from build123d import *

# Parameters (mm, degrees)
F1_R     = 63.5
F2_R     = 76.2
F4_R     = 26.2509
F5_DEPTH = 355.6
F6_R     = 25.4
F7_DEPTH = 95.25


with BuildPart() as f3:
    # F1 (on Top) → F3 section 0
    with BuildSketch(Plane.XY):
        Circle(F1_R)
    # F2 (on offset) → F3 section 1
    with BuildSketch(Plane.XY.offset(228.6)):
        Circle(F2_R)
    loft()

    # F4 (on Front) → F5 (join)
    with BuildSketch(Plane.XZ):
        with Locations((0, 151.5491)):
            Circle(F4_R)
    extrude(amount=F5_DEPTH)

    # F6 (on Front) → F7 (join)
    with BuildSketch(Plane.XZ):
        with Locations((0, 76.2)):
            Circle(F6_R)
    extrude(amount=-F7_DEPTH)


solid = f3.part
For this review, take the finished solid that the model builds, in its own axes (mm). A direction names the side the tool comes from. Give positions to 0.01 mm unless a question says otherwise; leave off trailing zeros. Order: outer loops, then holes, each group sorted by start corner. A loop starts at its lowest first (then second) coordinate and runs counter-clockwise, first axis right, second up. Notation, with made-up numbers: M 29,17 L 62,17 A15 ccw 62,36 Z; hole C -12.75,49.25 d4. An arc over 180 degrees is marked long. Answer in a Markdown table with one row per item. Add a question column.
(1) Consider section A-A on x = 0. State the section outline as (y, z) points, and give its area (3 significant figures).
(2) Consider section D-D on z = 86. State the section outline as (x, y) points, and give its area (3 significant figures).
(3) Consider section B-B on z = 111.5. State the section outline as (x, y) points.
(4) For faces 1 (the face through (-5.691, -209.179, 125.922)), 2 (the face through (0, -355.6, 152)), 3 (the face through (-5.506, 78.717, 51.404)), list the 3-axis set-ups (+Z, -Z, +X, -X, +Y, -Y) from which the entire face can be reached by the end or side of a thin tool; tool diameter is ignored.
(5) Wall thickness on probe 1 along Y at (x, z) = (35, 163); probe 2 along X at (y, z) = (-86, 157); probe 3 along Y at (x, z) = (27, 32): over which ranges is each line inside the solid? List them lowest first. Write a range as [from, to].
(6) Consider section C-C on y = -267. State the section outline as (x, z) points.
(7) For pin 1 (1 mm diameter, centred on x = 36, z = 40.5, fed in from +Y); pin 2 (8 mm diameter, centred on x = 58.5, z = 124, fed in from +Y); pin 3 (3 mm diameter, centred on y = 11.5, z = 62, fed in from +X), all flat-tipped, find the tip position at first contact; note any pin that passes through.
Evaluation:
| question | item | result |
|---|---|---|
| 1 | outline | M -355.6,125.3 L -70.46,125.3 L -63.5,0 L 63.5,0 L 66.32,50.8 L 95.25,50.8 L 95.25,101.6 L 69.14,101.6 L 76.2,228.6 L -76.2,228.6 L -73.38,177.8 L -355.6,177.8 Z |
| 1 | area | 48,200 mm^2 |
| 2 | outline | M -23.43,64.13 A68.28 ccw long 23.43,64.13 L 23.43,95.25 L -23.43,95.25 Z |
| 2 | area | 16,000 mm^2 |
| 3 | outline | C 0,0 d139.39 |
| 4 | face 1 | -Y |
| 4 | face 2 | +Z, -Z, +X, -X, -Y |
| 4 | face 3 | +Y |
| 5 | probe 1 | y = [-63.56, 63.56] |
| 5 | probe 2 | x = [-25.68, 25.68] |
| 5 | probe 3 | y = [-59.43, 59.43] |
| 6 | outline | C 0,151.55 d52.5 |
| 7 | pin 1 | stops at y = 55.34 |
| 7 | pin 2 | stops at y = 44.56 |
| 7 | pin 3 | stops at x = 66.21 |
